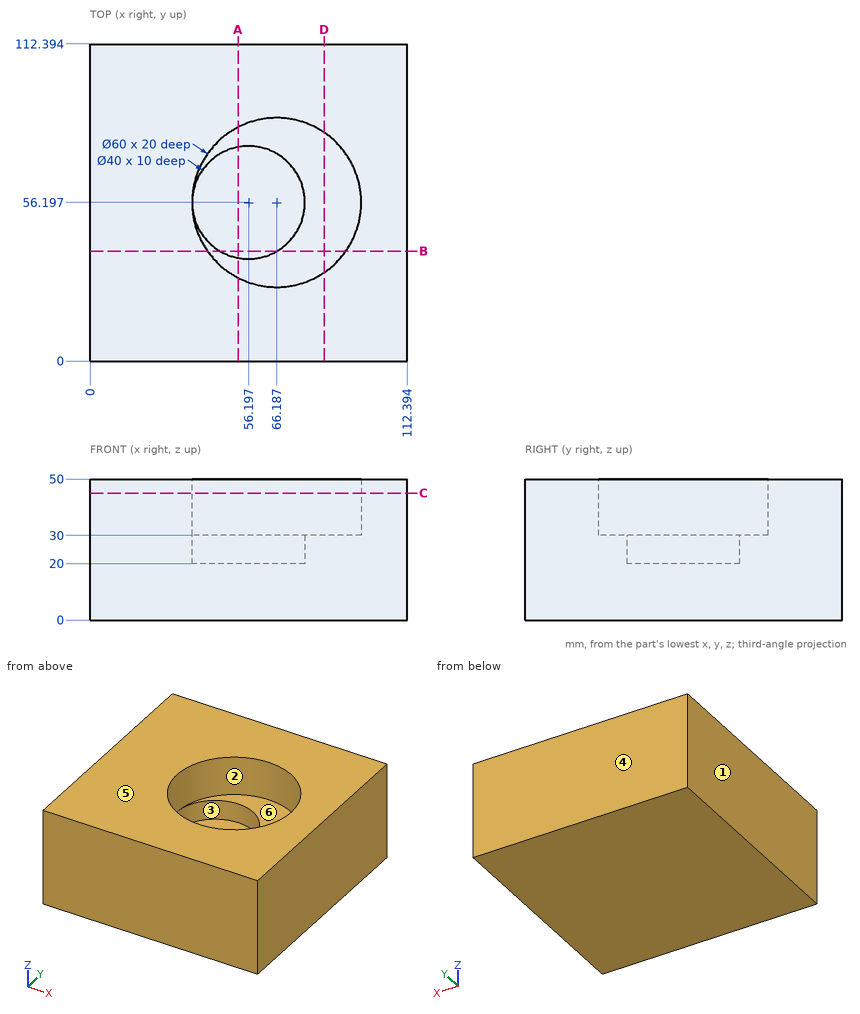
Geometry check sheet. Reference: drawing and pictorial views, mm from the part's lowest x, y, z. A direction names the side the tool comes from. Give positions to 0.01 mm unless a question says otherwise; leave off trailing zeros. Order: outer loops, then holes, each group sorted by start corner. A loop starts at its lowest first (then second) coordinate and runs counter-clockwise, first axis right, second up. Notation, with made-up numbers: M 65,24 L 93,24 A31 cw 93,51 Z; hole C 29.25,79 d10. An arc over 180 degrees is marked long. Return JSON: item names as keys, results as strings. Group by question number.
1) Go/stop test with a flat-tipped pin: pin 1 Ø20 at (x, y) = (65.5, 49.5) entering from +Z. Record where the tip stops, or that it passes through.
2) Access from +Z, -Z, +X, -X, +Y, -Y to the whole of each face (thin tool, end or side, straight path). Record for the marked faces 5 and 6.
3) Section check A-A on x = 52.5. Record the cut outline in (y, z), and give its area (3 significant figures).
4) Mould release check, pull along X, two halves, no side actions. Record for the marked faces 1, 2, 3 and 4: pulls with the +X half, pulls with the -X half, needs draft (parallel to the pull), parting line crosses it, or undercut.
5) Section check B-B on y = 39. Record the cut outline in (x, z) (1 decimal), and give its area (3 significant figures).
6) Scan lines: line 1 (Z direction, x = 55, y = 40); line 2 (Z direction, x = 44, y = 39); line 3 (Y direction, x = 68, z = 36). Record each from-to range of solid material in increasing order.
7) Section check D-D on x = 83. Record the cut outline in (y, z).
8) Section check C-C on z = 45. Record the cut outline in (x, y), and give its area (4 significant figures).
Answer block:
{
 "1": {"pin 1": "stops at z = 30"},
 "2": {"face 5": "+Z, +X, -X, +Y, -Y", "face 6": "+Z"},
 "3": {"outline": "M 0,0 L 112.39,0 L 112.39,50 L 82.89,50 L 82.89,30 L 75.85,30 L 75.85,20 L 36.54,20 L 36.54,30 L 29.5,30 L 29.5,50 L 0,50 Z", "area": "4,160 mm^2"},
 "4": {"face 1": "pulls with the -X half", "face 2": "undercut", "face 3": "undercut", "face 4": "needs draft"},
 "5": {"outline": "M 0,0 L 112.4,0 L 112.4,50 L 90.8,50 L 90.8,30 L 66.4,30 L 66.4,20 L 46,20 L 46,30 L 41.6,30 L 41.6,50 L 0,50 Z", "area": "4,430 mm^2"},
 "6": {"line 1": "z = 0 to 20", "line 2": "z = 0 to 30", "line 3": "y = 0 to 26.25, 86.14 to 112.39"},
 "7": {"outline": "M 0,0 L 112.39,0 L 112.39,50 L 81.04,50 L 81.04,30 L 31.35,30 L 31.35,50 L 0,50 Z"},
 "8": {"outline": "M 0,0 L 112.39,0 L 112.39,112.39 L 0,112.39 Z; hole C 66.19,56.2 d60", "area": "9,805 mm^2"}
}
